Autodesk Inventor part; units mm, degrees
ref_plane "YZ Plane" through (0, 0, 0) normal (1, 0, 0) x (0, 1, 0)
ref_plane "XZ Plane" through (0, 0, 0) normal (0, 1, 0) x (-1, 0, 0)
ref_plane "XY Plane" through (0, 0, 0) normal (0, 0, 1) x (1, 0, 0)
sketch "Boceto1" plane through (0, 0, 0) normal (0, 0, 1) x (1, 0, 0)
  line L0 (0, 0) -> (0, 500)
  line L1 (100, 500) -> (100, 0)
  line L2 (100, 0) -> (0, 0)
  line L3 (0, 500) -> (17.6777, 482.3223)
  line L4 (100, 500) -> (82.3223, 482.3223)
  line L5 (82.3223, 482.3223) -> (17.6777, 482.3223)
  line L6 (50, -100) -> (-150, -100)
revolve "Revolución1" add sketch "Boceto1" angle 360 about axis through (50, -100, 0) along (-1, 0, 0)
sketch "Boceto2" plane through (100, -100, 0) normal (1, 0, 0) x (0, 0, -1)
  circle A0 centre (0, 0) radius 100
  circle A1 centre (-350, 0) radius 37.5
  circle A2 centre (0, 350) radius 37.5
  circle A3 centre (350, 0) radius 37.5
  circle A4 centre (0, -350) radius 37.5
  point P0 (0, 100)
  dimension "d26" = 360
extrude "Extrusión1" cut sketch "Boceto2" against normal blind 100 contours A1 | A2 | A3 | A4
thicken "Engrosado1" operation add thickness 10 both sides no extend neighbours no toward (1, 0, 0) faces at (100, -364.9419, 262.9039)
thicken "Engrosado2" operation add thickness 10 both sides no extend neighbours no toward (-1, 0, 0) faces at (0, -364.9419, 262.9039)
sketch "Boceto3" plane through (110, -100, 0) normal (1, 0, 0) x (0, 0, -1)
  line L0 (-25, -96.8246) -> (-25, -125)
  line L1 (-25, -125) -> (25, -125)
  line L2 (25, -125) -> (25, -96.8246)
  circle A0 centre (0, 0) radius 100
  arc A1 (-25, -96.8246) -> (25, -96.8246) centre (0, 0) ccw
  point P0 (0, 100)
  point P1 (0, -100)
emboss "Repujado1" sketch "Boceto3" operation cut depth 120 direction (-1, 0, 0) contours A0 L2 L1 L0
properties part number "POLEA Pieza"
Input: part model. Units: mm. Frame: model coordinates. A direction names the side the tool comes from. Coordinates: 2 decimals unless noted, no trailing zeros. Write each loop counter-clockwise with the first axis right and the second up, starting at its lowest first coordinate (ties: lowest second). Pieces come first, ordered by that corner, then holes. Notation, with made-up numbers: M -10,43.5 L 35,43.5 A26 ccw 35,65.5 Z; hole C 22,-12.5 d6. An arc over 180 degrees is marked long. Answer as a JSON object with one key per item and string values. Group by question number.
(1) Mould query, pull axis X, two halves, no side actions, for faces 4 (the face through (110, 25, -8)), 5 (the face through (83.428, -226.476, -569.554)), 6 (the face through (51, -225, 0)). Classes: pulls with the +X half, pulls with the -X half, needs draft (parallel to the pull), parting line crosses it, or undercut.
(2) Section C-C on x = 38. Output: boundary loops of the cut face in (y, z).
(3) Section B-B on y = -100. Output: boundary loops of the cut face in (x, z).
(4) Set-up query: faces 1 (the face through (16.572, -226.476, 569.554)), 2 (the face through (51, -211, -25)), 3 (the face through (-10, 25, -8)). Return all of +Z, -Z, +X, -X, +Y, -Y with unobstructed straight access to the full face (end or side cutting, diameter ignored); none if empty.
(5) Ray query, line 1 along Y through (x, z) = (35, 0); line 2 along Z through (x, y) = (77.5, 267); line 3 along Y through (x, z) = (95, -41). Return the intervals inside material, ascending. Write a range as [from, to].
(6) Contact query for flat-ended pins moving along their axis: P1, Ø22.5, axis at x = 64.5, y = -209.5, coming from the -Z side; P2, Ø5, axis at x = 89, z = -329, coming from the -Y side; P3, Ø6, axis at x = 39, y = -218.5, coming from the -Z side. Output: stop coordinate, or through.
(7) Section A-A on z = 0. Output: boundary loops of the cut face in (x, y), plus the area to 3 significant figures.
Result set:
{
 "1": {"face 4": "pulls with the +X half", "face 5": "undercut", "face 6": "needs draft"},
 "2": {"outline": "C -100,0 d1164.64; hole C -450,0 d75; hole M -225,-25 L -196.82,-25 A100 ccw long -196.82,25 L -225,25 Z; hole C -100,-350 d75; hole C -100,350 d75; hole C 250,0 d75"},
 "3": {"outline": "M -10,-600 L 0,-600 L 17.68,-582.32 L 82.32,-582.32 L 100,-600 L 110,-600 L 110,-387.5 L -10,-387.5 Z; M -10,-312.5 L 110,-312.5 L 110,-100 L -10,-100 Z; M -10,100 L 110,100 L 110,312.5 L -10,312.5 Z; M -10,387.5 L 110,387.5 L 110,600 L 100,600 L 82.32,582.32 L 17.68,582.32 L 0,600 L -10,600 Z"},
 "4": {"face 1": "none", "face 2": "+X, -X", "face 3": "+Z, -Z, -X, +Y, -Y"},
 "5": {"line 1": "y = [-682.32, -487.5], [-412.5, -225], [0, 212.5], [287.5, 482.32]", "line 2": "z = [-452.12, -33.43], [33.43, 452.12]", "line 3": "y = [-693.59, -191.21], [-8.79, 493.59]"},
 "6": {"P1": "stops at z = -573.97", "P2": "stops at y = -591.99", "P3": "stops at z = -570.75"},
 "7": {"outline": "M -10,-700 L 0,-700 L 17.68,-682.32 L 82.32,-682.32 L 100,-700 L 110,-700 L 110,-487.5 L -10,-487.5 Z; M -10,-412.5 L 110,-412.5 L 110,-225 L -10,-225 Z; M -10,0 L 110,0 L 110,212.5 L -10,212.5 Z; M -10,287.5 L 110,287.5 L 110,500 L 100,500 L 82.32,482.32 L 17.68,482.32 L 0,500 L -10,500 Z", "area": "96,100 mm2"}
}
